```python
from build123d import *

# Parameters (mm, degrees)
F0_W     = 6
F0_H     = 2
F0_R     = 3
F0_W_2   = 5.1
F0_H_2   = 10.1
F1_DEPTH = 5
F0_W_3   = 460
F0_H_3   = 5
F2_DEPTH = 15


with BuildPart() as f1:
    # F0 (on Top) → F1 (new body)
    with BuildSketch(Plane.XY):
        with BuildLine():
            ThreePointArc((-80, -8), (-79.414214, -9.414214), (-78, -10))
            Line((-78, -10), (378, -10))
            ThreePointArc((378, -10), (379.414214, -9.414214), (380, -8))
            Line((380, -8), (380, 10))
            Line((380, 10), (-80, 10))
            Line((-80, 10), (-80, -8))
        make_face()
        with Locations((-60, -4)):
            Rectangle(F0_W, F0_H, mode=Mode.SUBTRACT)
        with Locations((80, -4)):
            Rectangle(F0_W, F0_H, mode=Mode.SUBTRACT)
        with Locations((-70, 0)):
            Circle(F0_R, mode=Mode.SUBTRACT)
        with Locations((70, 0)):
            Circle(F0_R, mode=Mode.SUBTRACT)
        with Locations((220, -4)):
            Rectangle(F0_W, F0_H, mode=Mode.SUBTRACT)
        with Locations((360, -4)):
            Rectangle(F0_W, F0_H, mode=Mode.SUBTRACT)
        with Locations((150, 0)):
            Rectangle(F0_W_2, F0_H_2, mode=Mode.SUBTRACT)
        with Locations((230, 0)):
            Circle(F0_R, mode=Mode.SUBTRACT)
        with Locations((370, 0)):
            Circle(F0_R, mode=Mode.SUBTRACT)
        with Locations((-60, 4)):
            Rectangle(F0_W, F0_H, mode=Mode.SUBTRACT)
        with Locations((80, 4)):
            Rectangle(F0_W, F0_H, mode=Mode.SUBTRACT)
        with Locations((220, 4)):
            Rectangle(F0_W, F0_H, mode=Mode.SUBTRACT)
        with Locations((360, 4)):
            Rectangle(F0_W, F0_H, mode=Mode.SUBTRACT)
    extrude(amount=F1_DEPTH)

    # F0 (on Top) → F2 (join)
    with BuildSketch(Plane.XY):
        with Locations((150, 12.5)):
            Rectangle(F0_W_3, F0_H_3)
    extrude(amount=F2_DEPTH)


solid = f1.part
```
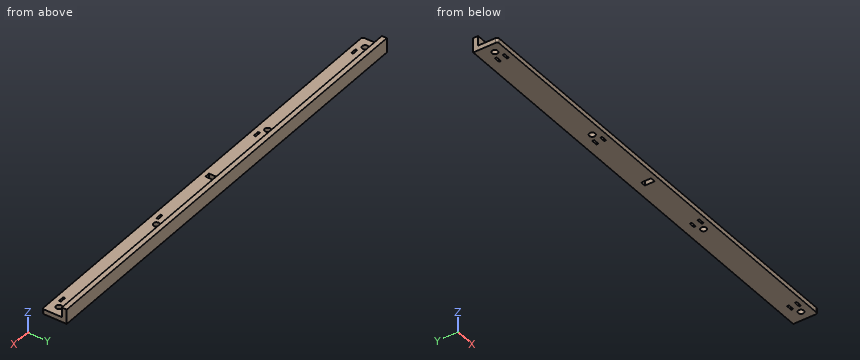
Model file for the job. Use its own axes, mm. Round coordinates to 2 decimals unless told otherwise and drop trailing zeros. Order: outer loops, then holes, each group sorted by start corner. A loop starts at its lowest first (then second) coordinate and runs counter-clockwise, first axis right, second up. Notation, with made-up numbers: (27, 65) -> (69, 65) arc R26 cw to (69, 103) -> close; hole circle Ø2 at (88.5, 67.25). An arc over 180 degrees is marked (long way). Use one line per item in the form item = value.
Item 1: Cut at B-B, the plane z = 11. Write the cut outline in (x, y).
Returned:
outline = (-80, 10) -> (380, 10) -> (380, 15) -> (-80, 15) -> close
Item 2: Drill centre lines: line 1 (X direction, y = 4, z = 3.75); line 2 (Y direction, x = -70, z = 3.15); line 3 (Z direction, x = 273, y = -6.25). Where is each one in solid material? Low to high.
Returned:
line_1 = -80 to -63, -57 to 77, 83 to 147.45, 152.55 to 217, 223 to 357, 363 to 380
line_2 = -10 to -3, 3 to 15
line_3 = 0 to 5
Item 3: Flat gauge pins, fed straight in: pin 1 Ø12 at (x, y) = (43, 2) entering from +Z; pin 2 Ø4 at (x, z) = (137, 10) entering from -Y. Where does each tip first touch, or does it go through?
Returned:
pin_1 = 5
pin_2 = 10
Item 4: Cut at A-A, the plane x = 342.5. Write the cut outline in (y, z).
Returned:
outline = (-10, 0) -> (15, 0) -> (15, 15) -> (10, 15) -> (10, 5) -> (-10, 5) -> close
